Check sheet for the modelled part. Datum: model origin and axes. Units: mm. Face numbers are marked on the shaded views. A direction names the side the tool comes from. Round coordinates to 2 decimals unless told otherwise and drop trailing zeros. Loops run counter-clockwise (first coordinate to the right, second up) from the corner with the lowest first, then second, coordinate; pieces in that order, holes last. Notation, with made-up numbers: (80, -29.75) -> (96, -29.75) arc R14 cw to (96, -7.75) -> close; hole circle Ø11 at (0.25, 14.5). An arc over 180 degrees is marked (long way). Use one line per item in the form item = value. Start each with the question number.
(1) Material ranges on probe 1 along X at (y, z) = (7, -6); probe 2 along Y at (x, z) = (2.25, 0); probe 3 along Y at (x, z) = (-1.15, 0), recorded low to high. Write a range as [from, to].
(2) Set-up check for the marked faces 4 and 5: record each of +Z, -Z, +X, -X, +Y, -Y from which the full face is reachable in a straight line by a thin tool's end or side.
(3) Sectioned sample at D-D (x = 2.5). Record the cut outline in (y, z), and give its area (3 significant figures).
(4) Draft check along Z on the marked faces 1, 2 and 3. Enter one of: released by +Z, released by -Z, zero draft, split by the parting line, or undercut.
(5) Sectioned sample at C-C (x = -2). Record the cut outline in (y, z), and give its area (3 significant figures).
(6) Go/stop test with flat-tipped pins: pin 1 (1.5 mm diameter, centred on x = -0.5, y = 7, fed in from -Z); pin 2 (1.5 mm diameter, centred on x = -0.5, y = -7.5, fed in from +Z); pin 3 (1 mm diameter, centred on x = 1.5, y = 3, fed in from -Z). Record where each tip stops, or that it passes through.
(7) Sectioned sample at A-A (y = 0). Record the cut outline in (x, z).
from build123d import *

# Parameters (mm, degrees)
SKETCH2_R          = 6
CUT_EXTRUDE1_DEPTH = 3


with BuildPart() as part:
    # Sketch1 → Revolve1 (revolve)
    with BuildSketch(Plane(origin=(0, 0, 0), x_dir=(1, 0, 0), z_dir=(0, 1, 0)), mode=Mode.PRIVATE) as revolve1_sk:
        with BuildLine():
            Line((-3.490371622, 9.75), (-2.490371622, 9.75))
            Line((-2.490371622, 9.75), (-2.490371622, 9.25))
            Line((-2.490371622, 9.25), (-0.990371622, 9.25))
            ThreePointArc((-0.990371622, 9.25), (0.259628378, 8.225245122), (1.509628378, 9.25))
            Line((1.509628378, 9.25), (3.259628378, 9.25))
            Line((3.259628378, 9.25), (3.259628378, 2))
            Line((3.259628378, 2), (-3.490371622, 2))
            Line((-3.490371622, 2), (-3.490371622, 9.75))
        make_face()
    revolve(revolve1_sk.sketch.rotate(Axis((-2.728053472, 0, 0), (1, 0, 0)), 180), axis=Axis((-2.728053472, 0, 0), (1, 0, 0)))

    # Sketch2 → Cut-Extrude1 (cut)
    with BuildSketch(Plane(origin=(3.259628378, 0, 0), x_dir=(0, 0, -1), z_dir=(1, 0, 0))):
        Circle(SKETCH2_R)
    extrude(amount=-CUT_EXTRUDE1_DEPTH, mode=Mode.SUBTRACT)


solid = part.part
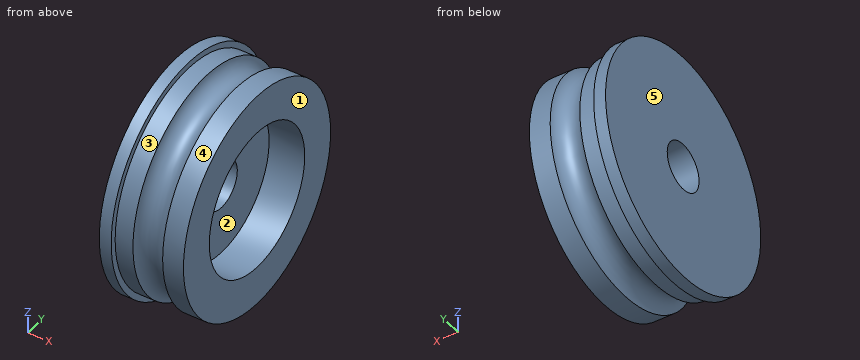
Checks:
q1.probe_1 = [-3.49, -0.98], [1.5, 3.26]
q1.probe_2 = [-9.25, -6], [6, 9.25]
q1.probe_3 = [-9.25, -2], [2, 9.25]
q2.face_4 = +X
q2.face_5 = +Z, -Z, -X, +Y, -Y
q3.outline = circle Ø18.5 at (0, 0); hole circle Ø12 at (0, 0)
q3.area = 156 mm2
q4.face_1 = zero draft
q4.face_2 = undercut
q4.face_3 = split by the parting line
q5.outline = circle Ø18.5 at (0, 0); hole circle Ø4 at (0, 0)
q5.area = 256 mm2
q6.pin_1 = -6.65
q6.pin_2 = 6.12
q6.pin_3 = -8.91
q7.outline = (-3.49, -9.75) -> (-2.49, -9.75) -> (-2.49, -9.25) -> (-0.99, -9.25) arc R1.27 cw to (1.51, -9.25) -> (3.26, -9.25) -> (3.26, -6) -> (0.26, -6) -> (0.26, -2) -> (-3.49, -2) -> close; (-3.49, 2) -> (0.26, 2) -> (0.26, 6) -> (3.26, 6) -> (3.26, 9.25) -> (1.51, 9.25) arc R1.27 cw to (-0.99, 9.25) -> (-2.49, 9.25) -> (-2.49, 9.75) -> (-3.49, 9.75) -> close
